Verification items for this drawing (mm, ordinates from the low corner). A direction names the side the tool comes from. Round coordinates to 2 decimals unless told otherwise and drop trailing zeros. Write item = value, one per line.
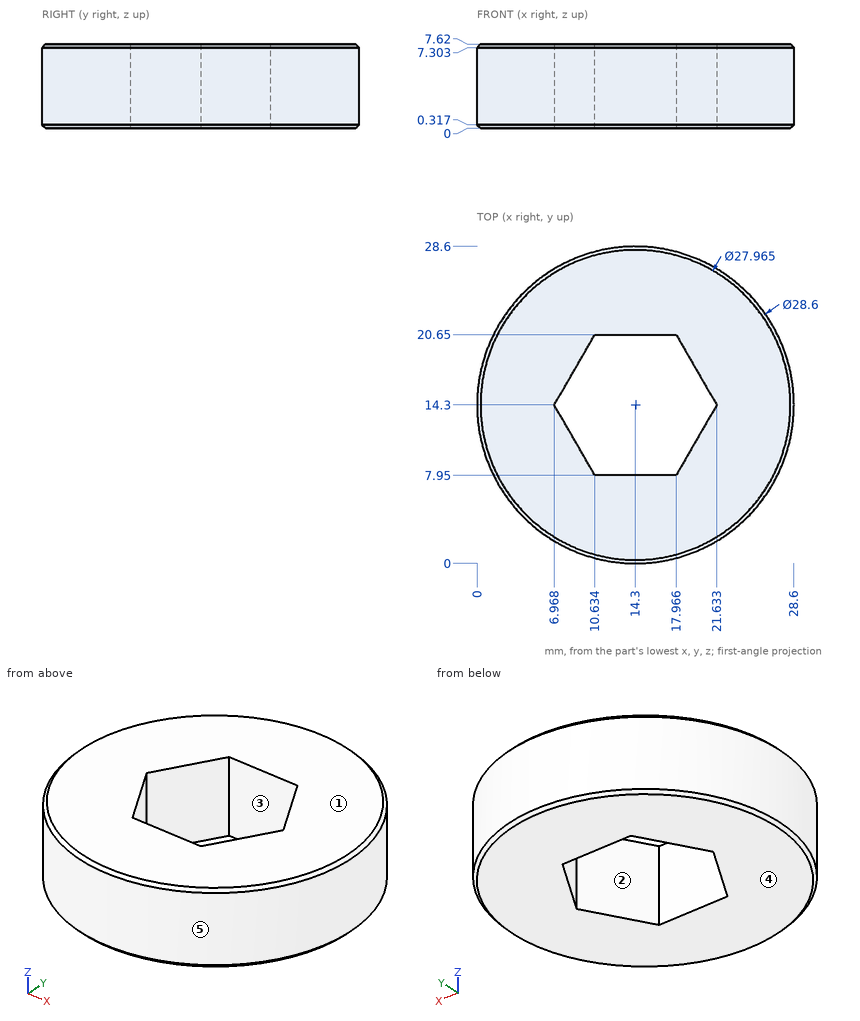
(1) Scan lines: L1, parallel to X at y = 8.5, z = 6.75 (1 decimal); L2, parallel to Y at x = 20, z = 0.5 (1 decimal); L3, parallel to X at y = 14.5, z = 5.75 (1 decimal). Record each from-to range of solid material in increasing order. Write a range as [from, to].
Answers follow:
L1 = [1.2, 10.3], [18.3, 27.4]
L2 = [1.2, 11.5], [17.1, 27.4]
L3 = [0, 7.1], [21.5, 28.6]
(2) Gauge pin test, flat ends, axial feed: pin 1 (1 mm diameter, centred on y = 13, z = 1.5, fed in from +X); pin 2 (5 mm diameter, centred on x = 15.5, y = 15, fed in from -Z). Record the tip position at first contact, or that the pin passes through.
Answers follow:
pin_1 = 28.58
pin_2 = through
(3) Set-up check for the marked faces 1 and 2: record each of +Z, -Z, +X, -X, +Y, -Y from which the full face is reachable in a straight line by a thin tool's end or side.
Answers follow:
face_1 = +Z, +X, -X, +Y, -Y
face_2 = +Z, -Z
(4) Mould release check, pull along Y, two halves, no side actions. Record for the marked faces 3, 4 and 5: pulls with the +Y half, pulls with the -Y half, needs draft (parallel to the pull), parting line crosses it, or undercut.
Answers follow:
face_3 = undercut
face_4 = needs draft
face_5 = parting line crosses it
